Can you work these out from the model? Positions are in its coordinate system, mm. A direction names the side the tool comes from. Coordinates: 2 decimals unless noted, no trailing zeros. Loops run counter-clockwise (first coordinate to the right, second up) from the corner with the lowest first, then second, coordinate; pieces in that order, holes last. Notation, with made-up numbers: M 58.5,40 L 116.5,40 A31 cw 116.5,72 Z; hole C 11,57 d11. An arc over 180 degrees is marked long. Answer as a JSON object with one key per item and string values. Group by question number.
Item 1: Suppose I cut it at D-D (x = -70). Write out the boundary of the cut face in (y, z), then the cut area to 3 significant figures.
Item 2: Suppose I cut it at A-A (y = 18.75). Write out the boundary of the cut face in (x, z).
Item 3: I'm going to push flat-ended pins straight in: pin 1 Ø4 at (y, z) = (28.72, 4.5) entering from +X; pin 2 Ø3.5 at (x, z) = (-70.5, 15.5) entering from +Y; pin 3 Ø1.5 at (y, z) = (13.5, 14.5) entering from +X; pin 4 Ø6 at (x, z) = (-67.5, 12) entering from -Y. Where does each tip first touch, or does it pass through?
Item 4: We'd pull the mould along Y, two halves only. Please class faces 1 (the flat face through (-64, 13.52, 8)), 2 (the flat face through (-29.53, 30.17, 1.46)), 3 (the flat face through (-63.7, 12.3, 12)), 4 (the flat face through (-73, 11.02, 15)): +Y half, -Y half, draft (parallel to the pull), parting line (faces both ways), or undercut.
Item 5: Suppose I cut it at C-C (y = 26.25). Write out the boundary of the cut face in (x, z).
Item 6: Which directions (+Z, -Z, +X, -X, +Y, -Y) give clear straight access to the entire face, cutting with the end or side of a thin tool? Please do faces 5 (the flat face through (-41.873, 21.465, 3.655)), 6 (the flat face through (-21.701, 17, 2)), 7 (the flat face through (-2, 12.02, 11)), 8 (the flat face through (-69.6, 16.8, 8)), 9 (the flat face through (-8, 21.5, 11.7)).
Item 7: If I drill on line 1 (X direction, y = 25.75, z = 1.25); line 2 (Y direction, x = -73, z = 10.25); line 3 (Z direction, x = -39, y = 12.25), over which ranges is the centre line in solid material (lowest first)?
```python
from build123d import *

# Parameters (mm, degrees)
CROQUIS1_W              = 88
CROQUIS1_H              = 11.7
SALIENTE_EXTRUIR1_DEPTH = 25
CORTAR_EXTRUIR1_DEPTH   = 11.7
CROQUIS4_W              = 7
CROQUIS4_H              = 6.7
CORTAR_EXTRUIR2_DEPTH   = 30
CROQUIS5_W              = 7
CROQUIS5_H              = 6.7
CORTAR_EXTRUIR3_DEPTH   = 30
CROQUIS6_W              = 5
CROQUIS6_H              = 6.7
CORTAR_EXTRUIR4_DEPTH   = 3
CROQUIS7_W              = 2.7
CROQUIS7_H              = 1
CORTAR_EXTRUIR5_DEPTH   = 30
CORTAR_EXTRUIR6_DEPTH   = 30
CROQUIS10_W             = 2.7
CROQUIS10_H             = 1
CORTAR_EXTRUIR7_DEPTH   = 30
CORTAR_EXTRUIR8_DEPTH   = 30
CROQUIS12_W             = 4
CROQUIS12_H             = 8.5
SALIENTE_EXTRUIR2_DEPTH = 10
CORTAR_EXTRUIR9_START   = -16.4
CROQUIS13_R             = 1.65
CORTAR_EXTRUIR9_DEPTH   = 16.4
CORTAR_EXTRUIR10_DEPTH  = 20
CROQUIS15_W             = 4
CROQUIS15_H             = 5.789985178
SALIENTE_EXTRUIR3_DEPTH = 1.292749
CORTAR_EXTRUIR11_START  = -16.4
CORTAR_EXTRUIR11_DEPTH  = 16.4
CROQUIS17_W             = 8.4
CROQUIS17_H             = 1.271995795
CORTAR_EXTRUIR12_DEPTH  = 20


with BuildPart() as part:
    # Croquis1 → Saliente-Extruir1 (new body)
    with BuildSketch(Plane.XY):
        with Locations((-35.700934579, 16.869626168)):
            Rectangle(CROQUIS1_W, CROQUIS1_H)
    extrude(amount=SALIENTE_EXTRUIR1_DEPTH)

    # Croquis3 → Cortar-Extruir1 (cut)
    with BuildSketch(Plane.XZ.offset(-11.019626168)):
        Polygon((-16.700934579, 3), (0.97673495, 20.67766953), (7.340695981, 14.313708499), (-6.973012518, 0), (8.299065421, 0), (8.299065421, 25), (-79.700934579, 25), (-79.700934579, 0), (-64.428856641, 0), (-78.74256514, 14.313708499), (-72.378604109, 20.67766953), (-54.700934579, 3), align=None)
    extrude(amount=-CORTAR_EXTRUIR1_DEPTH, mode=Mode.SUBTRACT)

    # Croquis4 → Cortar-Extruir2 (cut)
    with BuildSketch(Plane(origin=(-46.528136819, 0, 46.528136819), x_dir=(0.707106781186546, 0, 0.707106781186549), z_dir=(-0.707106781186549, 0, 0.707106781186546))):
        with Locations((-40.058081435, 16.869626168)):
            Rectangle(CROQUIS4_W, CROQUIS4_H)
    extrude(amount=-CORTAR_EXTRUIR2_DEPTH, mode=Mode.SUBTRACT)

    # Croquis5 → Cortar-Extruir3 (cut)
    with BuildSketch(Plane(origin=(10.82720224, 0, 10.82720224), x_dir=(0.7071067811865477, 0, -0.7071067811865475), z_dir=(0.7071067811865475, 0, 0.7071067811865477))):
        with Locations((-10.430664437, 16.869626168)):
            Rectangle(CROQUIS5_W, CROQUIS5_H)
    extrude(amount=-CORTAR_EXTRUIR3_DEPTH, mode=Mode.SUBTRACT)

    # Croquis6 → Cortar-Extruir4 (cut)
    with BuildSketch(Plane.XY.offset(3)):
        with Locations((-52.200934579, 16.869626168)):
            Rectangle(CROQUIS6_W, CROQUIS6_H)
        with Locations((-19.200934579, 16.869626168)):
            Rectangle(CROQUIS6_W, CROQUIS6_H)
    extrude(amount=-CORTAR_EXTRUIR4_DEPTH, mode=Mode.SUBTRACT)

    # Croquis7 → Cortar-Extruir5 (cut)
    with BuildSketch(Plane(origin=(-3.486506259, 0, 3.486506259), x_dir=(-0.7071067811865472, 0, -0.7071067811865479), z_dir=(0.7071067811865479, 0, -0.7071067811865472))):
        with Locations((-6.540655907, 11.519626168)):
            Rectangle(CROQUIS7_W, CROQUIS7_H)
        with Locations((-6.540655907, 22.219626168)):
            Rectangle(CROQUIS7_W, CROQUIS7_H)
    extrude(amount=-CORTAR_EXTRUIR5_DEPTH, mode=Mode.SUBTRACT)

    # Croquis9 → Cortar-Extruir6 (cut)
    with BuildSketch(Plane.XZ.offset(-12.019626168)):
        Polygon((0.183841731, 7.156854249), (2.093030041, 9.066042559), (1.672230345, 9.486842254), (-0.236957964, 7.577653945), align=None)
    extrude(amount=-CORTAR_EXTRUIR6_DEPTH, mode=Mode.SUBTRACT)

    # Croquis10 → Cortar-Extruir7 (cut)
    with BuildSketch(Plane(origin=(-32.21442832, 0, -32.21442832), x_dir=(-0.707106781186549, 0, 0.707106781186546), z_dir=(-0.707106781186546, 0, -0.707106781186549))):
        with Locations((57.029401778, 22.219626168)):
            Rectangle(CROQUIS10_W, CROQUIS10_H)
        with Locations((57.029401778, 11.519626168)):
            Rectangle(CROQUIS10_W, CROQUIS10_H)
    extrude(amount=-CORTAR_EXTRUIR7_DEPTH, mode=Mode.SUBTRACT)

    # Croquis11 → Cortar-Extruir8 (cut)
    with BuildSketch(Plane.XZ.offset(-12.019626168)):
        Polygon((-71.58571089, 7.156854249), (-70.878604109, 7.863961031), (-72.787792418, 9.77314934), (-73.494899199, 9.066042559), align=None)
    extrude(amount=-CORTAR_EXTRUIR8_DEPTH, mode=Mode.SUBTRACT)

    # Croquis12 → Saliente-Extruir2 (add)
    with BuildSketch(Plane(origin=(0, 22.719626168, 0), x_dir=(1, 0, 0), z_dir=(0, 1, 0))):
        with Locations((-29.500934579, -4.25)):
            Rectangle(CROQUIS12_W, CROQUIS12_H)
        with Locations((-41.900934579, -4.25)):
            Rectangle(CROQUIS12_W, CROQUIS12_H)
    extrude(amount=SALIENTE_EXTRUIR2_DEPTH)

    # Croquis13 → Cortar-Extruir9 (cut)
    with BuildSketch(Plane(origin=(-27.500934579, 0, 0), x_dir=(0, 0, -1), z_dir=(1, 0, 0)).offset(CORTAR_EXTRUIR9_START)):
        with Locations((-4.5, 28.719626168)):
            Circle(CROQUIS13_R)
        with BuildLine():
            Line((0, 27.719626168), (-2.971466884, 32.699888422))
            ThreePointArc((-2.971466884, 32.699888422), (-6.100596854, 31.91119471), (-8.46936188, 29.719746698))
            Line((-8.46936188, 29.719746698), (-4.292749227, 22.719626168))
            Line((-4.292749227, 22.719626168), (-8.5, 22.719626168))
            Line((-8.5, 22.719626168), (-8.5, 32.719626168))
            Line((-8.5, 32.719626168), (0, 32.719626168))
            Line((0, 32.719626168), (0, 27.719626168))
        make_face()
    extrude(amount=CORTAR_EXTRUIR9_DEPTH, mode=Mode.SUBTRACT)

    # Croquis14 → Cortar-Extruir10 (cut)
    with BuildSketch(Plane(origin=(-27.500934579, 0, 0), x_dir=(0, 0, -1), z_dir=(1, 0, 0))):
        with BuildLine():
            Line((-8.46936188, 29.719746698), (-7.269222305, 27.708278944))
            ThreePointArc((-7.269222305, 27.708278944), (-7.44017574, 30.019739431), (-6.100596854, 31.91119471))
            Line((-6.100596854, 31.91119471), (-7.548349231, 31.815598295))
            Line((-7.548349231, 31.815598295), (-8.46936188, 29.719746698))
        make_face()
    extrude(amount=-CORTAR_EXTRUIR10_DEPTH, mode=Mode.SUBTRACT)

    # Croquis15 → Saliente-Extruir3 (add)
    with BuildSketch(Plane.XY.offset(3)):
        with Locations((-41.900934579, 19.824633579)):
            Rectangle(CROQUIS15_W, CROQUIS15_H)
        with Locations((-29.500934579, 19.824633579)):
            Rectangle(CROQUIS15_W, CROQUIS15_H)
    extrude(amount=SALIENTE_EXTRUIR3_DEPTH)

    # Croquis16 → Cortar-Extruir11 (cut)
    with BuildSketch(Plane.ZY.offset(43.900934579).offset(CORTAR_EXTRUIR11_START)):
        Polygon((4.292749227, 22.719626168), (3, 20.175634578), (3, 16.92964099), (4.292749227, 16.92964099), align=None)
    extrude(amount=CORTAR_EXTRUIR11_DEPTH, mode=Mode.SUBTRACT)

    # Croquis17 → Cortar-Extruir12 (cut)
    with BuildSketch(Plane.XY.offset(3)):
        with Locations((-35.700934579, 22.083628271)):
            Rectangle(CROQUIS17_W, CROQUIS17_H)
    extrude(amount=-CORTAR_EXTRUIR12_DEPTH, mode=Mode.SUBTRACT)


solid = part.part
```
From the geometry:
{
 "1": {"outline": "M 11.02,5.57 L 22.72,5.57 L 22.72,8.74 L 21.72,8.74 L 21.72,12.56 L 22.72,12.56 L 22.72,18.3 L 20.22,18.3 L 20.22,8.4 L 13.52,8.4 L 13.52,18.3 L 11.02,18.3 L 11.02,12.56 L 12.02,12.56 L 12.02,8.74 L 11.02,8.74 Z", "area": "75.0 mm2"},
 "2": {"outline": "M -78.74,14.31 L -73.49,9.07 L -72.79,9.77 L -70.88,7.86 L -71.59,7.16 L -64.43,0 L -61.6,0 L -77.33,15.73 Z; M -49.7,0 L -21.7,0 L -21.7,3 L -49.7,3 Z; M -9.8,0 L -6.97,0 L 0.18,7.16 L -0.24,7.58 L 1.67,9.49 L 2.09,9.07 L 7.34,14.31 L 5.93,15.73 Z"},
 "3": {"pin 1": "x = -27.5", "pin 2": "y = 22.72", "pin 3": "x = 7.34", "pin 4": "y = 11.02"},
 "4": {"face 1": "undercut", "face 2": "+Y half", "face 3": "draft", "face 4": "-Y half"},
 "5": {"outline": "M -43.9,0 L -39.9,0 L -39.9,6.4 L -43.9,6.4 Z; M -31.5,0 L -27.5,0 L -27.5,6.4 L -31.5,6.4 Z"},
 "6": {"face 5": "+Z, -Y", "face 6": "+Z, -Z", "face 7": "-Y", "face 8": "+Z", "face 9": "+Z, +Y, -Y"},
 "7": {"line 1": "-43.9 to -39.9, -31.5 to -27.5", "line 2": "11.02 to 22.72", "line 3": "0 to 3"}
}
